The figure shows three views and two pictorial views of one solid part (mm, origin at its lowest corner). Answer the questions. Coordinates: 2 decimals unless noted, no trailing zeros. Order: outer loops, then holes, each group sorted by start corner. A loop starts at its lowest first (then second) coordinate and runs counter-clockwise, first axis right, second up.
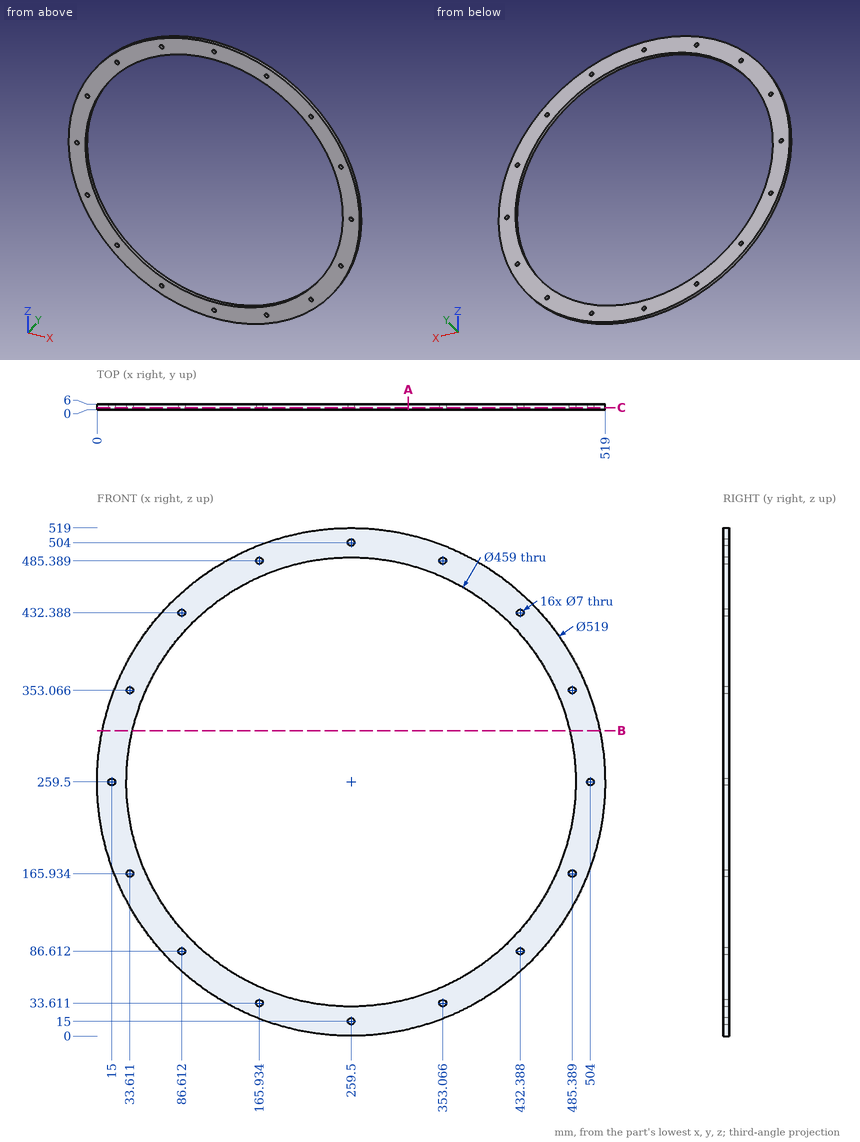
1) A cutting plane is placed at C-C, the plane y = 2.3. Count the separate pieces of the cut face and the enclosed holes in it, plus the area to 3 significant figures.
2) A cutting plane is placed at B-B, the plane z = 312. Write down the section's boundary in (x, y) (1 decimal).
3) Each of these flat-tipped pins is pushed along its axis until it touches: P1, Ø3, axis at y = 4.5, z = 185.5, coming from the -X side; P2, Ø1.5, axis at x = 74.5, y = 1, coming from the +Z side (1 decimal). Where does it stop, or does it pass through?
4) A cutting plane is placed at A-A, the plane x = 318. Write down the section's boundary in (y, z).
5) Straight lines are drawn through the part: probe 1 along Z at (x, y) = (50.5, 2.3) (1 decimal); probe 2 along X at (y, z) = (1.45, 351) (1 decimal); probe 3 along Z at (x, y) = (440.5, 4.15) (1 decimal). For each, find the intervals that lie inside material, in ascending order.
Working result:
1. separate pieces: 1
1. enclosed holes: 17
1. area: 45,500 mm2
2. outline: (5.4, 0) - (36.1, 0) - (36.1, 6) - (5.4, 6) - close; (482.9, 0) - (513.6, 0) - (513.6, 6) - (482.9, 6) - close
3. P1: stops at x = 10.33
3. P2: stops at z = 442.2
4. outline: (0, 6.68) - (6, 6.68) - (6, 37.58) - (0, 37.58) - close; (0, 481.42) - (6, 481.42) - (6, 512.32) - (0, 512.32) - close
5. probe 1: z = 105.7 to 164.7, 354.3 to 413.3
5. probe 2: x = 16.7 to 30.8, 36.4 to 49, 470 to 482.6, 488.2 to 502.3
5. probe 3: z = 73.5 to 118.4, 400.6 to 445.5
